from build123d import *

# Parameters (mm, degrees)
ESQUISSE1_W             = 26.5
ESQUISSE1_H             = 36
BOSS_EXTRU_1_DEPTH      = 1
ESQUISSE2_W             = 10
ESQUISSE2_H             = 2.5
BOSS_EXTRU_2_DEPTH      = 2.5
BOSS_EXTRU_3_DEPTH      = 5
BOSS_EXTRU_3_DEPTH_BACK = 4
ESQUISSE3_R             = 0.25
ESQUISSE4_W             = 1
ESQUISSE4_H             = 3
ESQUISSE4_H_2           = 2
ESQUISSE4_W_2           = 0.5
ESQUISSE4_H_3           = 1.5
ESQUISSE4_W_3           = 1.5
ESQUISSE4_H_4           = 1
BOSS_EXTRU_4_DEPTH      = 0.5
ESQUISSE5_R             = 2
BOSS_EXTRU_5_DEPTH      = 0.5
ESQUISSE6_R             = 2.25
BOSS_EXTRU_6_DEPTH      = 1.5
ESQUISSE7_W             = 15
ESQUISSE7_H             = 11.6
ESQUISSE7_W_2           = 2
ESQUISSE7_H_2           = 3
BOSS_EXTRU_7_DEPTH      = 2
ESQUISSE8_R             = 1.2
ESQUISSE8_R_2           = 1.05
ESQUISSE8_W             = 0.573696965
ESQUISSE8_H             = 1.577666654
ESQUISSE8_W_2           = 0.5
ESQUISSE8_H_2           = 1.5
ESQUISSE8_W_3           = 3
ESQUISSE8_H_3           = 1
BOSS_EXTRU_8_DEPTH      = 0.5


with BuildPart() as part:
    # Esquisse1 → Boss.-Extru.1 (new body)
    with BuildSketch(Plane.XY):
        with Locations((-13.25, 18)):
            Rectangle(ESQUISSE1_W, ESQUISSE1_H)
    extrude(amount=BOSS_EXTRU_1_DEPTH)

    # Esquisse2 → Boss.-Extru.2 (add)
    with BuildSketch(Plane.XY.offset(1)):
        with Locations((-13.25, 34.75)):
            Rectangle(ESQUISSE2_W, ESQUISSE2_H)
    extrude(amount=BOSS_EXTRU_2_DEPTH)

    # Esquisse3 → Boss.-Extru.3 (add, two sides: drawn at the far end of the back side and taken through both)
    with BuildSketch(Plane.XY.offset(3.5).offset(-BOSS_EXTRU_3_DEPTH_BACK)):
        with Locations((-17, 34.75)):
            Circle(ESQUISSE3_R)
        with Locations((-14.5, 34.75)):
            Circle(ESQUISSE3_R)
        with Locations((-12, 34.75)):
            Circle(ESQUISSE3_R)
        with Locations((-9.5, 34.75)):
            Circle(ESQUISSE3_R)
    extrude(amount=BOSS_EXTRU_3_DEPTH + BOSS_EXTRU_3_DEPTH_BACK)

    # Esquisse4 → Boss.-Extru.4 (add)
    with BuildSketch(Plane(origin=(0, 0, 0), x_dir=(-1, 0, 0), z_dir=(0, 0, -1))):
        with Locations((7.3, 31.311243574)):
            Rectangle(ESQUISSE4_W, ESQUISSE4_H)
        with Locations((9.3, 31.311243574)):
            Rectangle(ESQUISSE4_W, ESQUISSE4_H_2)
        with Locations((11.3, 31.311243574)):
            Rectangle(ESQUISSE4_W, ESQUISSE4_H_2)
        with Locations((13.05, 31.311243574)):
            Rectangle(ESQUISSE4_W_2, ESQUISSE4_H_3)
        with Locations((15.05, 31.311243574)):
            Rectangle(ESQUISSE4_W_3, ESQUISSE4_H_2)
        with Locations((17.05, 31.311243574)):
            Rectangle(ESQUISSE4_W_2, ESQUISSE4_H_4)
    extrude(amount=BOSS_EXTRU_4_DEPTH)

    # Esquisse5 → Boss.-Extru.5 (add)
    with BuildSketch(Plane(origin=(0, 0, 0), x_dir=(-1, 0, 0), z_dir=(0, 0, -1))):
        with Locations(Location((3, 27.5, 0), (0, 0, 180))):
            Circle(ESQUISSE5_R)
    extrude(amount=BOSS_EXTRU_5_DEPTH)

    # Esquisse6 → Boss.-Extru.6 (add)
    with BuildSketch(Plane(origin=(0, 0, -0.5), x_dir=(-1, 0, 0), z_dir=(0, 0, -1))):
        with Locations((3, 27.5)):
            Circle(ESQUISSE6_R)
    extrude(amount=BOSS_EXTRU_6_DEPTH)

    # Esquisse7 → Boss.-Extru.7 (add)
    with BuildSketch(Plane(origin=(0, 0, 0), x_dir=(-1, 0, 0), z_dir=(0, 0, -1))):
        with Locations((13, 16.3)):
            Rectangle(ESQUISSE7_W, ESQUISSE7_H)
        with Locations((2, 22.5)):
            Rectangle(ESQUISSE7_W_2, ESQUISSE7_H_2)
    extrude(amount=BOSS_EXTRU_7_DEPTH)

    # Esquisse8 → Boss.-Extru.8 (add)
    # profile 1 of 6: a face of its own
    with BuildSketch(Plane(origin=(0, 0, 0), x_dir=(-1, 0, 0), z_dir=(0, 0, -1))):
        with Locations(Location((17.5, 3, 0), (0, 0, 180))):
            Circle(ESQUISSE8_R)
        with Locations((17.5, 3)):
            Circle(ESQUISSE8_R_2, mode=Mode.SUBTRACT)
    # profile 2 of 6: a face of its own
    with BuildSketch(Plane(origin=(0, 0, 0), x_dir=(-1, 0, 0), z_dir=(0, 0, -1))):
        with Locations((3.927424315, 22.3983434)):
            Rectangle(ESQUISSE8_W, ESQUISSE8_H)
    # profile 3 of 6: a face of its own
    with BuildSketch(Plane(origin=(0, 0, 0), x_dir=(-1, 0, 0), z_dir=(0, 0, -1))):
        with Locations((1.404555649, 7.75)):
            Rectangle(ESQUISSE8_W_2, ESQUISSE8_H_2)
    # profile 4 of 6: a face of its own
    with BuildSketch(Plane(origin=(0, 0, 0), x_dir=(-1, 0, 0), z_dir=(0, 0, -1))):
        with Locations((2.886606143, 7.75)):
            Rectangle(ESQUISSE8_W_2, ESQUISSE8_H_2)
    # profile 5 of 6: a face of its own
    with BuildSketch(Plane(origin=(0, 0, 0), x_dir=(-1, 0, 0), z_dir=(0, 0, -1))):
        with Locations((15.25, 7.25)):
            Rectangle(ESQUISSE8_W_2, ESQUISSE8_H_2)
    # profile 6 of 6: a face of its own
    with BuildSketch(Plane(origin=(0, 0, 0), x_dir=(-1, 0, 0), z_dir=(0, 0, -1))):
        with Locations((17.7, 6.5)):
            Rectangle(ESQUISSE8_W_3, ESQUISSE8_H_3)
    extrude(amount=BOSS_EXTRU_8_DEPTH)


solid = part.part
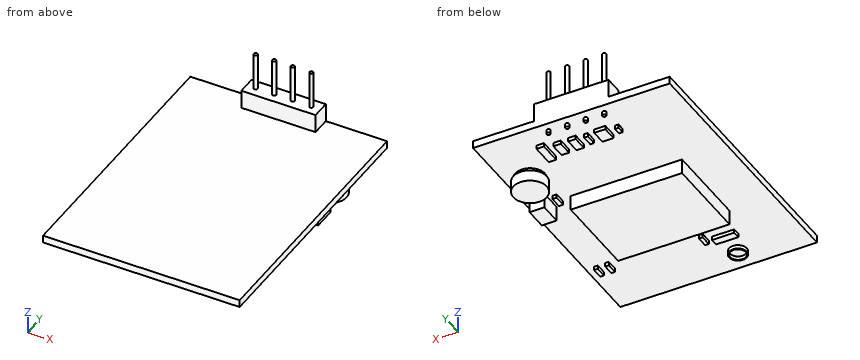
Work out the finished part from the listing and answer in its coordinate system (mm). Round coordinates to 2 decimals unless told otherwise and drop trailing zeros. Order: outer loops, then holes, each group sorted by start corner. A loop starts at its lowest first (then second) coordinate and runs counter-clockwise, first axis right, second up. Notation, with made-up numbers: M 13,1 L 35,1 A12 cw 35,13 Z; hole C 21,71 d4. An arc over 180 degrees is marked long. Put each result on its own line as item: value. Start each with the question number.
Q1. Section C-C, the plane z = 7.25 is taken. Write down the section's boundary in (x, y), and give its area (3 significant figures).
Q2. Straight lines are drawn through the part: L1, parallel to Z at x = -1.5, y = 23.5; L2, parallel to X at y = 34, z = 2.75; L3, parallel to Z at x = -3.5, y = 2.5. For each, find the intervals that lie inside material, in ascending order. Write a range as [from, to].
Q3. Section A-A, the plane y = 27.5 is taken. Write down the section's boundary in (x, z), and give its area (4 significant figures).
Q4. Flat-ended cylindrical pins translate along their axes: pin 1 (0.6 mm diameter, centred on y = 6.5, z = -0.5, fed in from +X); pin 2 (12 mm diameter, centred on x = -19, y = 10, fed in from +Z); pin 3 (2 mm diameter, centred on x = -2, z = -1.5, fed in from +Y). Find the tip coordinate at first contact, or state that the pin passes through.
Q5. Section D-D, the plane y = 3 is taken. Write down the section's boundary in (x, z), and give its area (4 significant figures).
Q6. Section B-B, the plane x = -20 is taken. Write down the section's boundary in (y, z).
Findings below:
1. outline: C -17,34.75 d0.5; C -14.5,34.75 d0.5; C -12,34.75 d0.5; C -9.5,34.75 d0.5
1. area: 0.785 mm^2
2. L1: z = [-2, 1]
2. L2: x = [-18.25, -8.25]
2. L3: z = [0, 1]
3. outline: M -26.5,0 L -5,0 L -5,-0.5 L -5.25,-0.5 L -5.25,-2 L -0.75,-2 L -0.75,-0.5 L -1,-0.5 L -1,0 L 0,0 L 0,1 L -26.5,1 Z
3. area: 35.25 mm^2
4. pin 1: stops at x = -15
4. pin 2: stops at z = 1
4. pin 3: stops at y = 29.75
5. outline: M -26.5,0 L -18.7,0 L -18.7,-0.5 L -18.55,-0.5 L -18.55,0 L -16.45,0 L -16.45,-0.5 L -16.3,-0.5 L -16.3,0 L 0,0 L 0,1 L -26.5,1 Z
5. area: 26.65 mm^2
6. outline: M 0,0 L 10.5,0 L 10.5,-2 L 22.1,-2 L 22.1,0 L 36,0 L 36,1 L 0,1 Z
